Check sheet for the modelled part. Datum: model origin and axes. Units: mm. A direction names the side the tool comes from. Give positions to 0.01 mm unless a question says otherwise; leave off trailing zeros. Write each loop counter-clockwise with the first axis right and the second up, starting at its lowest first coordinate (ties: lowest second). Pieces come first, ordered by that corner, then holes. Notation, with made-up numbers: (-19, 0) - (-11, 0) arc R28 ccw to (-11, 30) - close; hole circle Ø8 at (34.25, -13.75). An arc over 180 degrees is marked (long way). Return JSON: item names as keys, results as strings. Group by question number.
```python
from build123d import *

# Parameters (mm, degrees)
F0_W      = 42.2
F0_H      = 42.2
F0_R      = 2.5
F1_DEPTH  = 33.3
F2_SIZE   = 5
F3_DEPTH  = 20
F4_R      = 11
F4_R_2    = 4.5
F5_DEPTH  = 2
F6_R      = 1.25
F7_DEPTH  = 5
F9_W      = 50.7564134896
F9_H      = 50.1955691725
F10_DEPTH = 16
F11_R     = 2
F12_R     = 9.5
F13_DEPTH = 12.25
F14_R     = 4
F15_DEPTH = 12.7
F16_R     = 1
F17_W     = 1
F17_H     = 1


with BuildPart() as f1:
    # F0 (on Front) → F1 (new body)
    with BuildSketch(Plane.XZ):
        Rectangle(F0_W, F0_H)
        Circle(F0_R, mode=Mode.SUBTRACT)
        Circle(F0_R)
    extrude(amount=-F1_DEPTH)

    # F2
    f2_edges = [f1.edges().sort_by_distance(p)[0] for p in [
        (21.1, 16.65, 21.1),
        (-21.1, 16.65, 21.1),
        (21.1, 16.65, -21.1),
        (-21.1, 16.65, -21.1),
    ]]
    chamfer(f2_edges, length=F2_SIZE)

    # F0 (on Front) → F3 (join)
    with BuildSketch(Plane.XZ):
        Circle(F0_R)
    extrude(amount=F3_DEPTH)

    # F4 (on face) → F5 (join)
    with BuildSketch(Plane.XZ):
        Circle(F4_R)
        Circle(F4_R_2, mode=Mode.SUBTRACT)
    extrude(amount=F5_DEPTH)

    # F6 (on face) → F7 (cut)
    with BuildSketch(Plane.XZ):
        with Locations((-15.5, 15.5)):
            Circle(F6_R)
        with Locations((-15.5, -15.5)):
            Circle(F6_R)
        with Locations((15.5, -15.5)):
            Circle(F6_R)
        with Locations((15.5, 15.5)):
            Circle(F6_R)
    extrude(amount=-F7_DEPTH, mode=Mode.SUBTRACT)

    # F9 (on offset) → F10 (cut)
    with BuildSketch(Plane.XZ.offset(-8)):
        with Locations((0.5305930972, 0.0707069412)):
            Rectangle(F9_W, F9_H)
        Polygon((-14.3372583002, 20.6), (0, 20.6), (14.3372583002, 20.6), (20.6, 14.3372583002), (20.6, 0), (20.6, -14.3372583002), (14.3372583002, -20.6), (0, -20.6), (-14.3372583002, -20.6), (-20.6, -14.3372583002), (-20.6, 0), (-20.6, 14.3372583002), align=None, mode=Mode.SUBTRACT)
    extrude(amount=-F10_DEPTH, mode=Mode.SUBTRACT)

    # F11
    f11_edges = [f1.edges().sort_by_distance(p)[0] for p in [
        (20.6, 16, 14.337258),
        (14.337258, 16, 20.6),
        (-14.337258, 16, 20.6),
        (-20.6, 16, 14.337258),
        (-20.6, 16, -14.337258),
        (-14.337258, 16, -20.6),
        (20.6, 16, -14.337258),
        (14.337258, 16, -20.6),
    ]]
    fillet(f11_edges, radius=F11_R)

    # F12 (on face) → F13 (join, symmetric)
    with BuildSketch(Plane.XZ.offset(20)):
        Circle(F12_R)
    extrude(amount=F13_DEPTH, both=True)

    # F14 (on face) → F15 (cut)
    with BuildSketch(Plane.XZ.offset(32.25)):
        Circle(F14_R)
    extrude(amount=-F15_DEPTH, mode=Mode.SUBTRACT)

    # F16
    f16_edges = [f1.edges().sort_by_distance(p)[0] for p in [
        (-9.5, -32.25, 0),
        (-9.5, -7.75, 0),
        (-4, -32.25, 0),
    ]]
    fillet(f16_edges, radius=F16_R)

    # F17 (on Right) → F18 (revolve, cut)
    with BuildSketch(Plane.YZ):
        with Locations((-16.55, 9)):
            Rectangle(F17_W, F17_H)
        with Locations((-18.55, 9)):
            Rectangle(F17_W, F17_H)
        with Locations((-20.55, 9)):
            Rectangle(F17_W, F17_H)
        with Locations((-22.55, 9)):
            Rectangle(F17_W, F17_H)
    revolve(axis=Axis((0, -8.7481234223, 0), (0, 1, 0)), mode=Mode.SUBTRACT)


solid = f1.part
```
Item 1: Section check B-B on x = -12. Record the cut outline in (y, z).
Item 2: Access from +Z, -Z, +X, -X, +Y, -Y to the whole of each face (thin tool, end or side, straight path). Record for faces 1 (the face through (17, 8, -19)), 2 (the face through (15.34, 2.46, -14.26)), 3 (the face through (20.444, 16.112, 14.284)), 4 (the face through (-14.284, 16.112, 20.444)).
Item 3: Section check A-A on y = -1. Record the cut outline in (x, z).
Item 4: Mould release check, pull along X, two halves, no side actions. Record for faces 5 (the face through (-16, 5, -15)), 6 (the face through (-8.4, -20.05, 2.2)), 7 (the face through (14.264, 16.112, -20.452)): +X half, -X half, draft (parallel to the pull), parting line (faces both ways), or undercut.
Item 5: Section check D-D on y = -25.5. Record the cut outline in (x, z).
Item 6: Depth check by flat-ended pin: pin 1 (4 mm diameter, centred on x = 15.5, z = -15.5, fed in from -Y); pin 2 (5 mm diameter, centred on y = 17, z = 2.5, fed in from +X); pin 3 (1.5 mm diameter, centred on x = 9.5, z = -6, fed in from -Y). Enter the tip coordinate at first touch or a pass-through.
Item 7: Material ranges on line 1 along Z through (x, y) = (15.5, 3.95); line 2 along Z through (x, y) = (0, -27.25); line 3 along Y through (x, z) = (19, 17.5), recorded low to high. Write a range as from..to.
Item 8: Section check C-C on y = 19. Record the cut outline in (x, z), plus the area to 3 significant figures.
Reply:
{
 "1": {"outline": "(0, -21.1) - (8, -21.1) - (8, -20.6) - (24, -20.6) - (24, -21.1) - (33.3, -21.1) - (33.3, 21.1) - (24, 21.1) - (24, 20.6) - (8, 20.6) - (8, 21.1) - (0, 21.1) - close"},
 "2": {"face 1": "none", "face 2": "-Y", "face 3": "+Z, +X", "face 4": "+Z, -X"},
 "3": {"outline": "circle Ø22 at (0, 0); circle Ø5 at (0, 0); hole circle Ø9 at (0, 0)"},
 "4": {"face 5": "undercut", "face 6": "draft", "face 7": "+X half"},
 "5": {"outline": "circle Ø19 at (0, 0); hole circle Ø8 at (0, 0)"},
 "6": {"pin 1": "y = 0", "pin 2": "x = 20.6", "pin 3": "y = -2"},
 "7": {"line 1": "-21.1..-16.75, -14.25..14.25, 16.75..21.1", "line 2": "-9.5..-4, 4..9.5", "line 3": "0..8, 24..33.3"},
 "8": {"outline": "(-20.6, -13.51) arc R2 ccw to (-20.01, -14.92) - (-14.92, -20.01) arc R2 ccw to (-13.51, -20.6) - (13.51, -20.6) arc R2 ccw to (14.92, -20.01) - (20.01, -14.92) arc R2 ccw to (20.6, -13.51) - (20.6, 13.51) arc R2 ccw to (20.01, 14.92) - (14.92, 20.01) arc R2 ccw to (13.51, 20.6) - (-13.51, 20.6) arc R2 ccw to (-14.92, 20.01) - (-20.01, 14.92) arc R2 ccw to (-20.6, 13.51) - close", "area": "1,620 mm²"}
}
